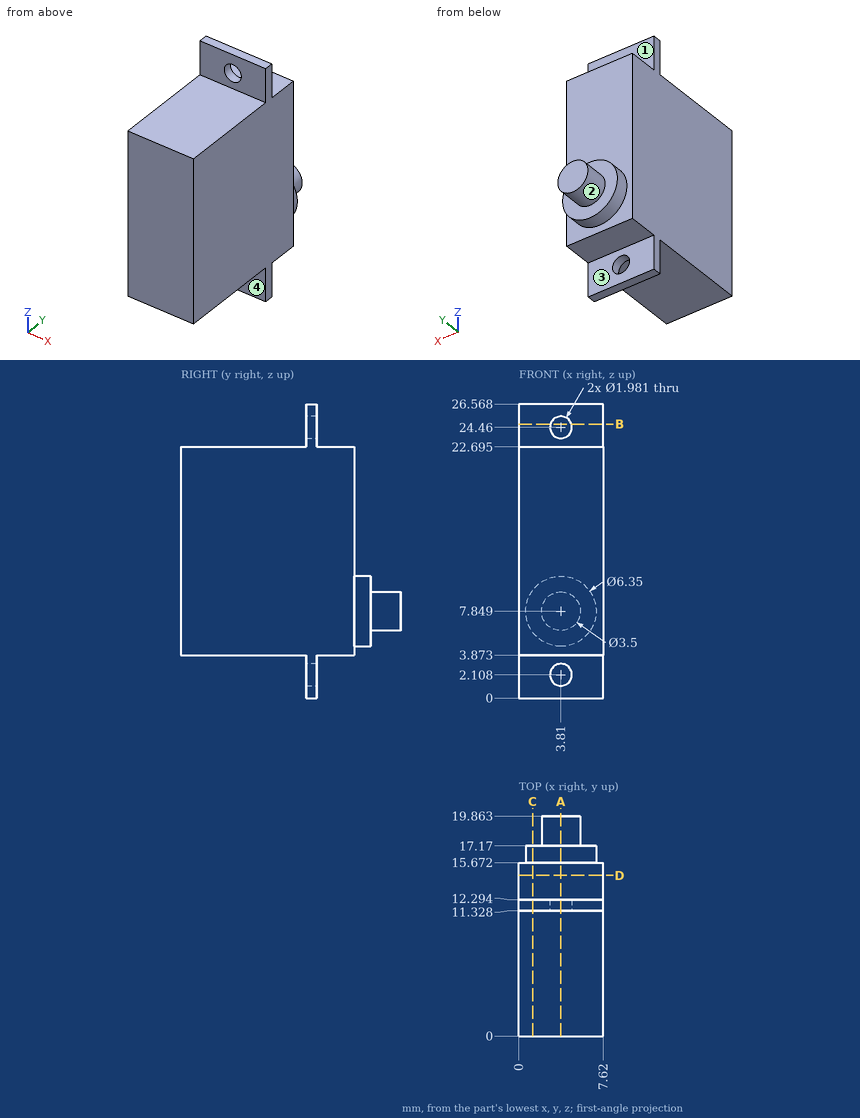
Print and shaded views of the part. All mm, measured from the part's lowest x, y and z. A direction names the side the tool comes from. Give positions to 0.01 mm unless a question says otherwise; leave off trailing zeros. Write each loop counter-clockwise with the first axis right and the second up, starting at its lowest first coordinate (ties: lowest second). Pieces come first, ordered by that corner, then holes. Notation, with made-up numbers: M 19.25,76 L 63.25,76 A9 cw 63.25,82 Z; hole C 22.25,33.5 d5. An arc over 180 degrees is marked long. Use a Markdown table: item, result.
1) Cut at D-D (y = 14.5). List the corners of the cut face in (x, z) (1 decimal).
Responses:
| item | result |
|---|---|
| outline | M 0,3.9 L 7.6,3.9 L 7.6,22.7 L 0,22.7 Z |
2) Cut at A-A (x = 3.81). Give the number of separate pieces and of enclosed holes in the cut face.
Responses:
| item | result |
|---|---|
| separate pieces | 3 |
| enclosed holes | 0 |
3) Drill centre lines: line 1 (Y direction, x = 6, z = 2); line 2 (Z direction, x = 5.75, y = 12.5) (1 decimal); line 3 (Y direction, x = 6.5, z = 4.25). Where is each one in solid material? Low to high. Write a range as from..to.
Responses:
| item | result |
|---|---|
| line 1 | y = 11.33..12.29 |
| line 2 | z = 3.9..22.7 |
| line 3 | y = 0..15.67 |
4) Cut at B-B (z = 24.75). List the corners of the cut face in (x, y).
Responses:
| item | result |
|---|---|
| outline | M 0,11.33 L 2.86,11.33 L 2.86,12.29 L 0,12.29 Z; M 4.76,11.33 L 7.62,11.33 L 7.62,12.29 L 4.76,12.29 Z |
5) Tool access for the marked faces 1, 2, 3 and 4: list every direction of +Z, -Z, +X, -X, +Y, -Y with a clear straight run to the whole face (end or side of a thin tool).
Responses:
| item | result |
|---|---|
| face 1 | +Z, +X, -X, +Y |
| face 2 | +Y |
| face 3 | -Z, +X, -X, +Y |
| face 4 | -Z, +X, -X, -Y |
6) Pin check, flat tips, straight feed: pin 1 (3.5 mm diameter, centred on x = 5, y = 14.5, fed in from -Z); pin 2 (2 mm diameter, centred on x = 2.5, y = 10, fed in from +Z) (1 decimal); pin 3 (4 mm diameter, centred on x = 5.5, z = 13, fed in from +Y); pin 4 (1.8 mm diameter, centred on x = 3.81, z = 2.11, fed in from +Y). Stop position of each tip, or through.
Responses:
| item | result |
|---|---|
| pin 1 | stops at z = 3.87 |
| pin 2 | stops at z = 22.7 |
| pin 3 | stops at y = 15.67 |
| pin 4 | passes through |
7) Cut at C-C (x = 1.25). List the corners of the cut face in (y, z) (1 decimal).
Responses:
| item | result |
|---|---|
| outline | M 0,3.9 L 11.3,3.9 L 11.3,0 L 12.3,0 L 12.3,3.9 L 15.7,3.9 L 15.7,6 L 17.2,6 L 17.2,9.7 L 15.7,9.7 L 15.7,22.7 L 12.3,22.7 L 12.3,26.6 L 11.3,26.6 L 11.3,22.7 L 0,22.7 Z |
